Source: CAD feature listing. Evaluate the final solid. Frame: model axes, mm. A direction names the side the tool comes from. Round coordinates to 2 decimals unless told otherwise and drop trailing zeros. Write each loop counter-clockwise with the first axis right and the second up, starting at its lowest first coordinate (ties: lowest second). Pieces come first, ordered by that corner, then holes. Notation, with made-up numbers: (47, 45) -> (54, 45) arc R23 cw to (54, 77) -> close; hole circle Ø5 at (-20, 38.25). An arc over 180 degrees is marked (long way). Put each result on its own line as item: value.
```python
from build123d import *

# Parameters (mm, degrees)
F1_DEPTH = 3.2
F0_R     = 2.1
F2_DEPTH = 7
F3_R     = 2.3


with BuildPart() as f1:
    # F0 (on Top) → F1 (new body)
    with BuildSketch(Plane.XY):
        with BuildLine():
            Line((8.5, 0), (8.5, 2))
            ThreePointArc((8.5, 2), (3.9038059223, 3.9038059223), (2, 8.5))
            Line((2, 8.5), (0, 8.5))
            Line((0, 8.5), (-2, 8.5))
            ThreePointArc((-2, 8.5), (-3.9038059223, 3.9038059223), (-8.5, 2))
            Line((-8.5, 2), (-8.5, 0))
            Line((-8.5, 0), (-8.5, -2))
            ThreePointArc((-8.5, -2), (-3.9038059223, -3.9038059223), (-2, -8.5))
            Line((-2, -8.5), (0, -8.5))
            Line((0, -8.5), (2, -8.5))
            ThreePointArc((2, -8.5), (3.9038059223, -3.9038059223), (8.5, -2))
            Line((8.5, -2), (8.5, 0))
        make_face()
        Polygon((0, 4.0414518843), (3.5, 2.0207259422), (3.5, -2.0207259422), (0, -4.0414518843), (-3.5, -2.0207259422), (-3.5, 2.0207259422), align=None, mode=Mode.SUBTRACT)
    extrude(amount=F1_DEPTH)

    # F0 (on Top) → F2 (join)
    with BuildSketch(Plane.XY):
        with BuildLine():
            Line((8.5, 0), (8.5, 2))
            ThreePointArc((8.5, 2), (3.9038059223, 3.9038059223), (2, 8.5))
            Line((2, 8.5), (0, 8.5))
            Line((0, 8.5), (-2, 8.5))
            ThreePointArc((-2, 8.5), (-3.9038059223, 3.9038059223), (-8.5, 2))
            Line((-8.5, 2), (-8.5, 0))
            Line((-8.5, 0), (-8.5, -2))
            ThreePointArc((-8.5, -2), (-3.9038059223, -3.9038059223), (-2, -8.5))
            Line((-2, -8.5), (0, -8.5))
            Line((0, -8.5), (2, -8.5))
            ThreePointArc((2, -8.5), (3.9038059223, -3.9038059223), (8.5, -2))
            Line((8.5, -2), (8.5, 0))
        make_face()
        Polygon((0, 4.0414518843), (3.5, 2.0207259422), (3.5, -2.0207259422), (0, -4.0414518843), (-3.5, -2.0207259422), (-3.5, 2.0207259422), align=None, mode=Mode.SUBTRACT)
        Polygon((3.5, -2.0207259422), (3.5, 2.0207259422), (0, 4.0414518843), (-3.5, 2.0207259422), (-3.5, -2.0207259422), (0, -4.0414518843), align=None)
        Circle(F0_R, mode=Mode.SUBTRACT)
    extrude(amount=-F2_DEPTH)

    # F3
    f3_edges = [f1.edges().sort_by_distance(p)[0] for p in [
        (8.5, 2, -1.9),
        (8.5, -2, -1.9),
        (2, -8.5, -1.9),
        (2, 8.5, -1.9),
        (-2, 8.5, -1.9),
        (-8.5, 2, -1.9),
        (-8.5, -2, -1.9),
        (-2, -8.5, -1.9),
    ]]
    fillet(f3_edges, radius=F3_R)


solid = f1.part
```
Q1. Pin query (flat end, axial travel): pin 1 (4 mm diameter, centred on x = -5.5, y = -3, fed in from -Z); pin 2 (3 mm diameter, centred on x = 4, z = 2, fed in from +Y); pin 3 (5 mm diameter, centred on x = 0, y = 0, fed in from +Z); pin 4 (2 mm diameter, centred on x = -1.5, z = -3.5, fed in from -Y). Return the tip coordinate at first contact, or that it passes through.
Ans:
pin 1: stops at z = -7
pin 2: stops at y = 6
pin 3: stops at z = 0
pin 4: stops at y = -8.45
Q2. Cut plane C-C on x = -0.75. Output: boundary loops of the cut face in (y, z).
Ans:
outline: (-8.38, -7) -> (-1.96, -7) -> (-1.96, 0) -> (-3.61, 0) -> (-3.61, 3.2) -> (-8.38, 3.2) -> close; (1.96, -7) -> (8.38, -7) -> (8.38, 3.2) -> (3.61, 3.2) -> (3.61, 0) -> (1.96, 0) -> close
Q3. Cut plane B-B on y = -0.5. Output: boundary loops of the cut face in (x, z).
Ans:
outline: (-8.45, -7) -> (-2.04, -7) -> (-2.04, 0) -> (-3.5, 0) -> (-3.5, 3.2) -> (-8.45, 3.2) -> close; (2.04, -7) -> (8.45, -7) -> (8.45, 3.2) -> (3.5, 3.2) -> (3.5, 0) -> (2.04, 0) -> close
Q4. Material intervals for line 1 (Y direction, x = 0, z = -5); line 2 (X direction, y = 0.25, z = -0.25); line 3 (Z direction, x = -0.25, y = -2.75), sorted ascending. Write a range as [from, to].
Ans:
line 1: y = [-8.5, -2.1], [2.1, 8.5]
line 2: x = [-8.49, -2.09], [2.09, 8.49]
line 3: z = [-7, 0]
Q5. Draft query along X for faces 1 (the cylindrical face through (-1.387, -8.039, -1.971)), 2 (the cylindrical face through (1.42, -8.014, -1.971)), 3 (the cylindrical face through (2.003, 0.631, -3.451)). Return one class per face: +X half, -X half, draft (parallel to the pull), parting line (faces both ways), or undercut.
Ans:
face 1: -X half
face 2: +X half
face 3: undercut
Q6. Reachability of faces 4 (the flat face through (1.8, -3, 1.6)), 5 (the cylindrical face through (-8.014, -1.42, -1.829)) from +Z, -Z, +X, -X, +Y, -Y: full face, straight path, thin tool, end or side. Return the list, or none.
Ans:
face 4: +Z
face 5: +Z, -Z, -X, -Y
Q7. Cut plane D-D on x = -6. Output: boundary loops of the cut face in (y, z), and give its area (3 significant figures).
Ans:
outline: (-2.5, -7) -> (2.5, -7) -> (2.5, 3.2) -> (-2.5, 3.2) -> close
area: 51.0 mm^2
